```python
from build123d import *

# Parameters (mm, degrees)
SKETCH1_R           = 5
SKETCH1_R_2         = 1.5
BOSS_EXTRUDE1_DEPTH = 2
SKETCH3_R           = 1.55
CUT_EXTRUDE1_DEPTH  = 10


with BuildPart() as part:
    # Sketch1 → Boss-Extrude1 (new body)
    with BuildSketch(Plane.XY):
        with BuildLine():
            Line((-3.75, 16), (-3.75, 11.75))
            ThreePointArc((-3.75, 11.75), (-6.093145751, 6.093145751), (-11.75, 3.75))
            Line((-11.75, 3.75), (-16, 3.75))
            ThreePointArc((-16, 3.75), (-19.75, 0), (-16, -3.75))
            Line((-16, -3.75), (-11.75, -3.75))
            ThreePointArc((-11.75, -3.75), (-6.093145751, -6.093145751), (-3.75, -11.75))
            Line((-3.75, -11.75), (-3.75, -16))
            ThreePointArc((-3.75, -16), (0, -19.75), (3.75, -16))
            Line((3.75, -16), (3.75, -11.75))
            ThreePointArc((3.75, -11.75), (6.093145751, -6.093145751), (11.75, -3.75))
            Line((11.75, -3.75), (16, -3.75))
            ThreePointArc((16, -3.75), (19.75, 0), (16, 3.75))
            Line((16, 3.75), (11.75, 3.75))
            ThreePointArc((11.75, 3.75), (6.093145751, 6.093145751), (3.75, 11.75))
            Line((3.75, 11.75), (3.75, 16))
            ThreePointArc((3.75, 16), (0, 19.75), (-3.75, 16))
        make_face()
        Circle(SKETCH1_R, mode=Mode.SUBTRACT)
        with Locations((-16, 0)):
            Circle(SKETCH1_R_2, mode=Mode.SUBTRACT)
        with Locations((0, 16)):
            Circle(SKETCH1_R_2, mode=Mode.SUBTRACT)
        with Locations((16, 0)):
            Circle(SKETCH1_R_2, mode=Mode.SUBTRACT)
        with Locations((0, -16)):
            Circle(SKETCH1_R_2, mode=Mode.SUBTRACT)
    extrude(amount=BOSS_EXTRUDE1_DEPTH)

    # Sketch3 → Cut-Extrude1 (cut)
    with BuildSketch(Plane(origin=(0, 0, 0), x_dir=(-1, 0, 0), z_dir=(0, 0, -1))):
        with BuildLine():
            ThreePointArc((9.49046875, -0.425444362), (9.5, 0), (9.49046875, 0.425444362))
            ThreePointArc((9.49046875, 0.425444362), (6.45, 0), (9.49046875, -0.425444362))
        make_face()
        with Locations((0, 9.5)):
            Circle(SKETCH3_R)
        with Locations((0, -9.5)):
            Circle(SKETCH3_R)
        with Locations((-8, 0)):
            Circle(SKETCH3_R)
    extrude(amount=-CUT_EXTRUDE1_DEPTH, mode=Mode.SUBTRACT)


solid = part.part
```
Can you work these out from the model? Positions are in its coordinate system, mm. A direction names the side the tool comes from. Coordinates: 2 decimals unless noted, no trailing zeros. Loops run counter-clockwise (first coordinate to the right, second up) from the corner with the lowest first, then second, coordinate; pieces in that order, holes last. Notation, with made-up numbers: (58, 13) - (81, 13) arc R15 cw to (81, 32) - close; hole circle Ø1 at (0.25, 89.5). An arc over 180 degrees is marked (long way). Use a Markdown table: item, result.
Item 1: I want a section at D-D on y = 12.5. Please give me the cut outline in (x, z), and give its area (3 significant figures).
Numbers:
| item | result |
|---|---|
| outline | (-3.75, 0) - (3.75, 0) - (3.75, 2) - (-3.75, 2) - close |
| area | 15.0 mm2 |
Item 2: We'd pull the mould along X, two halves only. Please class faces 6 (the face through (0.336, 7.987, 0.986)), 7 (the face through (-6.156, -6.031, 0.986)), 8 (the face through (6.156, 6.031, 0.986)), 9 (the face through (-14, -3.75, 1)): released by +X, released by -X, zero draft, split by the parting line, or undercut.
Numbers:
| item | result |
|---|---|
| face 6 | undercut |
| face 7 | released by -X |
| face 8 | released by +X |
| face 9 | zero draft |
Item 3: I want a section at B-B on z = 0.6. Give the number of separate pieces and of enclosed holes in the cut face, and give its area (3 significant figures).
Numbers:
| item | result |
|---|---|
| separate pieces | 1 |
| enclosed holes | 9 |
| area | 430 mm2 |
Item 4: Will these pins go through, and if not, where does the flat tip stop? pin 1 (1 mm diameter, centred on y = -13.5, z = 1, fed in from -X); pin 2 (5 mm diameter, centred on x = -16, y = 0, fed in from +Z); pin 3 (0.6 mm diameter, centred on x = 13.5, z = 1, fed in from -Y); pin 4 (1 mm diameter, centred on x = -13.5, z = 1, fed in from +Y).
Numbers:
| item | result |
|---|---|
| pin 1 | stops at x = -3.75 |
| pin 2 | stops at z = 2 |
| pin 3 | stops at y = -3.75 |
| pin 4 | stops at y = 3.75 |
Item 5: I want a section at A-A on y = 3. Please give me the cut outline in (x, z), and give its area (3 significant figures).
Numbers:
| item | result |
|---|---|
| outline | (-18.25, 0) - (-4, 0) - (-4, 2) - (-18.25, 2) - close; (4, 0) - (18.25, 0) - (18.25, 2) - (4, 2) - close |
| area | 57.0 mm2 |
Item 6: I want a section at C-C on x = 8. Please give me the cut outline in (y, z).
Numbers:
| item | result |
|---|---|
| outline | (-4.68, 0) - (-1.55, 0) - (-1.55, 2) - (-4.68, 2) - close; (1.55, 0) - (4.68, 0) - (4.68, 2) - (1.55, 2) - close |
Item 7: If I drill on probe 1 along Y at (x, z) = (0, 1.3); probe 2 along Y at (x, z) = (-16, 1.1); probe 3 along X at (y, z) = (13, 1.9), over which ranges is the centre line in solid material (lowest first)? Write a range as from..to.
Numbers:
| item | result |
|---|---|
| probe 1 | y = -19.75..-17.5, -14.5..-11.05, -7.95..-5, 5..7.95, 11.05..14.5, 17.5..19.75 |
| probe 2 | y = -3.75..-1.5, 1.5..3.75 |
| probe 3 | x = -3.75..3.75 |
Item 8: For faces 1 (the face through (-14, 3.75, 1)), 2 (the face through (-9.5, 0, 1)), 3 (the face through (3.75, 14, 1)), 4 (the face through (14, -3.75, 1)), 5 (the face through (-3.75, -14, 1)), which set-ups out of +Z, -Z, +X, -X, +Y, -Y let a thin tool reach every point of the face, with its end or its side?
Numbers:
| item | result |
|---|---|
| face 1 | +Z, -Z, -X, +Y |
| face 2 | +Z, -Z |
| face 3 | +Z, -Z, +X, +Y |
| face 4 | +Z, -Z, +X, -Y |
| face 5 | +Z, -Z, -X, -Y |
